Verification items for the finished model (mm, model axes). Give positions to 0.01 mm unless a question says otherwise; leave off trailing zeros. Order: outer loops, then holes, each group sorted by start corner. A loop starts at its lowest first (then second) coordinate and runs counter-clockwise, first axis right, second up. Notation, with made-up numbers: (-39.75, 55.5) - (-34.75, 55.5) arc R28 cw to (-34.75, 88.5) - close; hole circle Ø9 at (80.25, 64.25). An arc over 180 degrees is marked (long way). Answer as a JSON object with one key per item and string values. Group by question number.
(1) Depth check by flat-ended pin: pin 1 Ø5.5 at (x, y) = (0, 0) entering from -Z; pin 2 Ø4 at (x, y) = (-2, 0.5) entering from -Z. Enter the tip coordinate at first touch or a pass-through.
(2) Mould release check, pull along X, two halves, no side actions. Record for faces 1 (the face through (5.2, 0, 2.3)), 2 (the face through (-3, 0, 0)), 3 (the face through (0, -5, 0)), 4 (the face through (-4.35, -2.465, 0.035)): +X half, -X half, draft (parallel to the pull), parting line (faces both ways), or undercut.
(3) Section check B-B (z = -2.1). Record the boundary of the cut face in (x, y), then the cut area to 3 significant figures.
(4) Section check A-A (z = 0.25). Record the boundary of the cut face in (x, y), then the cut area to 3 significant figures.
(5) Thickness scan on line 1 (Y direction, x = -0.5, z = 1.1); line 2 (Y direction, x = 1.25, z = 0.1); line 3 (X direction, y = -0.75, z = -1.75). Record the ranges inside material, lowest first.
```python
from build123d import *

# Parameters (mm, degrees)
F0_R     = 3
F1_DEPTH = 2.5


with BuildPart() as f1:
    # F0 (on Top) → F1 (new body, symmetric)
    with BuildSketch(Plane.XY):
        Polygon((2.886751, 5), (-2.886751, 5), (-5.773503, 0), (-2.886751, -5), (2.886751, -5), (5.773503, 0), align=None)
        Circle(F0_R, mode=Mode.SUBTRACT)
    extrude(amount=F1_DEPTH, both=True)

    # F2 (on Front) → F3 (revolve, cut)
    with BuildSketch(Plane.XZ):
        Polygon((-5.773503, 2.5), (-5.773503, 1.726497), (-5, 2.5), align=None)
        Polygon((-5, -2.5), (-5.773503, -1.726497), (-5.773503, -2.5), align=None)
    revolve(axis=Axis((0, 0, -0.060454), (0, 0, -1)), mode=Mode.SUBTRACT)


solid = f1.part
```
Solutions:
{
 "1": {"pin 1": "passes through", "pin 2": "stops at z = -2.5"},
 "2": {"face 1": "+X half", "face 2": "undercut", "face 3": "draft", "face 4": "-X half"},
 "3": {"outline": "(-5.35, -0.73) - (-3.31, -4.27) arc R5.4 ccw to (-2.04, -5) - (2.04, -5) arc R5.4 ccw to (3.31, -4.27) - (5.35, -0.73) arc R5.4 ccw to (5.35, 0.73) - (3.31, 4.27) arc R5.4 ccw to (2.04, 5) - (-2.04, 5) arc R5.4 ccw to (-3.31, 4.27) - (-5.35, 0.73) arc R5.4 ccw to start; hole circle Ø6 at (0, 0)", "area": "56.8 mm2"},
 "4": {"outline": "(-5.77, 0) - (-2.89, -5) - (2.89, -5) - (5.77, 0) - (2.89, 5) - (-2.89, 5) - close; hole circle Ø6 at (0, 0)", "area": "58.3 mm2"},
 "5": {"line 1": "y = -5 to -2.96, 2.96 to 5", "line 2": "y = -5 to -2.73, 2.73 to 5", "line 3": "x = -5.34 to -2.9, 2.9 to 5.34"}
}
